from build123d import *

# Parameters (mm, degrees)
SKETCH_1_W                    = 280
SKETCH_1_H                    = 35
EXTRUDE_1_DEPTH               = 26
SKETCH_3_R                    = 9
CUT_EXTRUDE_1_DEPTH           = 36
SKETCH_4_W                    = 25
SKETCH_4_H                    = 26
CUT_EXTRUDE_2_DEPTH           = 1
HOLE_WIZARD_M4_1_D            = 3.3
HOLE_WIZARD_M4_1_DEPTH        = 10.1
HOLE_WIZARD_M4_1_TIP          = 0.991420021
SKETCH_7_W                    = 220
SKETCH_7_H                    = 15
CUT_EXTRUDE_3_DEPTH           = 27
SKETCH_8_W                    = 40
SKETCH_8_H                    = 26
EXTRUDE_2_DEPTH               = 35
SKETCH_15_W                   = 58.430685067
SKETCH_15_H                   = 44.376242578
CUT_EXTRUDE_7_DEPTH           = 3
SKETCH_17_W                   = 40
SKETCH_17_H                   = 26
EXTRUDE_4_DEPTH               = 30
SKETCH_18_W                   = 20
SKETCH_18_H                   = 62
CUT_EXTRUDE_8_DEPTH           = 27
SKETCH_19_W                   = 30
SKETCH_19_H                   = 26
CUT_EXTRUDE_11_DEPTH          = 7
HOLE_WIZARD_M5_1_2_AT_2_COUNT = 2
HOLE_WIZARD_M5_1_2_AT_2_PITCH = 30
CHAMFER_1_SIZE                = 5
CHAMFER_1_SIZE2               = 2.886751346
CHAMFER_2_SIZE                = 5
CHAMFER_2_SIZE2               = 2.886751346
SKETCH_25_R                   = 2.5
CUT_EXTRUDE_12_DEPTH          = 21.0000001
SKETCH_26_R                   = 2.5
CUT_EXTRUDE_13_DEPTH          = 161.0000001
SKETCH_27_R                   = 5
CUT_EXTRUDE_14_DEPTH          = 83
SKETCH_28_R                   = 7
CUT_EXTRUDE_15_DEPTH          = 6
SKETCH_31_W                   = 13
SKETCH_31_H                   = 28
CUT_EXTRUDE_16_DEPTH          = 1
HOLE_WIZARD_M3_1_D            = 2.5
HOLE_WIZARD_M3_1_DEPTH        = 7.5
HOLE_WIZARD_M3_1_TIP          = 0.751075774
SKETCH_34_W                   = 5
SKETCH_34_H                   = 8
CUT_EXTRUDE_17_DEPTH          = 27


with BuildPart() as part:
    # 草图1 → 凸台-拉伸1 (new body)
    with BuildSketch(Plane.XY):
        with Locations((140, 17.5)):
            Rectangle(SKETCH_1_W, SKETCH_1_H)
    extrude(amount=EXTRUDE_1_DEPTH)

    # 草图3 → 切除-拉伸1 (cut, through all)
    with BuildSketch(Plane.XZ):
        with Locations((17, 13)):
            Circle(SKETCH_3_R)
        with Locations((263, 13)):
            Circle(SKETCH_3_R)
    extrude(amount=-CUT_EXTRUDE_1_DEPTH, mode=Mode.SUBTRACT)

    # 草图4 → 切除-拉伸2 (cut)
    with BuildSketch(Plane(origin=(0, 35, 0), x_dir=(1, 0, 0), z_dir=(0, 1, 0))):
        with Locations((140, -13)):
            Rectangle(SKETCH_4_W, SKETCH_4_H)
    extrude(amount=-CUT_EXTRUDE_2_DEPTH, mode=Mode.SUBTRACT)

    # M4 螺纹孔1
    with Locations(Plane(origin=(0, 34, 0), x_dir=(1, 0, 0), z_dir=(0, 1, 0))):
        with Locations((146, -21.5), (134, -21.5), (146, -4.5), (133.546958493, -4.5)):
            Hole(HOLE_WIZARD_M4_1_D / 2, depth=HOLE_WIZARD_M4_1_DEPTH)
            with Locations((0, 0, -(HOLE_WIZARD_M4_1_DEPTH + HOLE_WIZARD_M4_1_TIP / 2))):  # 118° drill point
                Cone(0, HOLE_WIZARD_M4_1_D / 2, HOLE_WIZARD_M4_1_TIP, mode=Mode.SUBTRACT)

    # 草图7 → 切除-拉伸3 (cut, through all)
    with BuildSketch(Plane.XY.offset(26)):
        with Locations((140, 7.5)):
            Rectangle(SKETCH_7_W, SKETCH_7_H)
    extrude(amount=-CUT_EXTRUDE_3_DEPTH, mode=Mode.SUBTRACT)

    # 草图8 → 凸台-拉伸2 (add)
    with BuildSketch(Plane.XZ.offset(-15)):
        with Locations((140, 13)):
            Rectangle(SKETCH_8_W, SKETCH_8_H)
    extrude(amount=EXTRUDE_2_DEPTH)

    # 草图15 → 切除-拉伸7 (cut)
    with BuildSketch(Plane.XZ.offset(20)):
        with Locations((130.784657466, 3.811878711)):
            Rectangle(SKETCH_15_W, SKETCH_15_H)
    extrude(amount=-CUT_EXTRUDE_7_DEPTH, mode=Mode.SUBTRACT)

    # 草图17 → 凸台-拉伸4 (add)
    with BuildSketch(Plane.XZ.offset(17)):
        with Locations((140, 13)):
            Rectangle(SKETCH_17_W, SKETCH_17_H)
    extrude(amount=EXTRUDE_4_DEPTH)

    # 草图18 → 切除-拉伸8 (cut, through all)
    with BuildSketch(Plane(origin=(0, 0, 0), x_dir=(-1, 0, 0), z_dir=(0, 0, -1))):
        with Locations((-140, -16)):
            Rectangle(SKETCH_18_W, SKETCH_18_H)
    extrude(amount=-CUT_EXTRUDE_8_DEPTH, mode=Mode.SUBTRACT)

    # 草图19 → 切除-拉伸11 (cut)
    with BuildSketch(Plane.XZ):
        with Locations((265, 13)):
            Rectangle(SKETCH_19_W, SKETCH_19_H)
        with Locations((15, 13)):
            Rectangle(SKETCH_19_W, SKETCH_19_H)
    extrude(amount=-CUT_EXTRUDE_11_DEPTH, mode=Mode.SUBTRACT)

    # 草图21 → Hole Wizard M5 _1 (revolve, cut)
    with BuildSketch(Plane(origin=(280, 21, 13), x_dir=(0, 0, -1), z_dir=(0, 1, 0))):
        Polygon((0, 0), (0, 13.6618073), (2.1, 12.4), (2.1, 0), align=None)
    hole_wizard_m5_1 = revolve(axis=Axis((286.35, 21, 13), (-1, 0, 0)), mode=Mode.SUBTRACT)

    # 镜向1: Hole Wizard M5 _1 across plane
    add(hole_wizard_m5_1.mirror(Plane.ZY.offset(-140)), mode=Mode.SUBTRACT)

    # 草图24 → Hole Wizard M5 _1 2 (revolve, cut)
    with BuildSketch(Plane(origin=(160, -35, 10), x_dir=(0, 0, -1), z_dir=(0, 1, 0))):
        Polygon((0, 0), (0, 14.052366702), (2.75, 12.4), (2.75, 5.4), (5, 5.4), (5, 0), align=None)
    hole_wizard_m5_1_2 = revolve(axis=Axis((166.35, -35, 10), (-1, 0, 0)), mode=Mode.SUBTRACT)

    # Hole Wizard M5 _1 2 at 2: Hole Wizard M5 _1 2 ×2
    with Locations(*[(0, i * HOLE_WIZARD_M5_1_2_AT_2_PITCH, 0) for i in range(1, HOLE_WIZARD_M5_1_2_AT_2_COUNT)]):
        add(hole_wizard_m5_1_2, mode=Mode.SUBTRACT)

    # 倒角1
    chamfer_1_edges = [part.edges().sort_by_distance(p)[0] for p in [
        (150, -16, 0),
    ]]
    chamfer_1_side = [part.faces().sort_by_distance(p)[0] for p in [
        (150, -15.878511748, 13.091116189),
    ]]
    chamfer(chamfer_1_edges, length=CHAMFER_1_SIZE, length2=CHAMFER_1_SIZE2, reference=chamfer_1_side[0])

    # 倒角2
    chamfer_2_edges = [part.edges().sort_by_distance(p)[0] for p in [
        (130, -16, 0),
    ]]
    chamfer_2_side = [part.faces().sort_by_distance(p)[0] for p in [
        (130, -16, 13),
    ]]
    chamfer(chamfer_2_edges, length=CHAMFER_2_SIZE, length2=CHAMFER_2_SIZE2, reference=chamfer_2_side[0])

    # 镜向2: Hole Wizard M5 _1 2 across plane
    add(hole_wizard_m5_1_2.mirror(Plane.ZY.offset(-140)), mode=Mode.SUBTRACT)

    # 镜向2 copy 1 sketch → 镜向2 copy 1 (revolve, cut)
    with BuildSketch(Plane(origin=(120, -5, 10), x_dir=(0, 0, -1), z_dir=(0, 1, 0))):
        Polygon((0, 0), (0, -14.052366702), (2.75, -12.4), (2.75, -5.4), (5, -5.4), (5, 0), align=None)
    revolve(axis=Axis((113.65, -5, 10), (-1, 0, 0)), mode=Mode.SUBTRACT)

    # 草图25 → 切除-拉伸12 (cut, through all)
    with BuildSketch(Plane.XZ.offset(-15)):
        with Locations((140, 20.49725583)):
            Circle(SKETCH_25_R)
    extrude(amount=-CUT_EXTRUDE_12_DEPTH, mode=Mode.SUBTRACT)

    # 草图26 → 切除-拉伸13 (cut, through all)
    with BuildSketch(Plane.ZY.offset(-120)):
        with Locations((10, -20)):
            Circle(SKETCH_26_R)
    extrude(amount=-CUT_EXTRUDE_13_DEPTH, mode=Mode.SUBTRACT)

    # 草图27 → 切除-拉伸14 (cut, through all)
    with BuildSketch(Plane(origin=(0, 35, 0), x_dir=(1, 0, 0), z_dir=(0, 1, 0))):
        with Locations((196.4, -13)):
            Circle(SKETCH_27_R)
        with Locations((83.6, -13)):
            Circle(SKETCH_27_R)
    extrude(amount=-CUT_EXTRUDE_14_DEPTH, mode=Mode.SUBTRACT)

    # 草图28 → 切除-拉伸15 (cut)
    with BuildSketch(Plane(origin=(0, 35, 0), x_dir=(1, 0, 0), z_dir=(0, 1, 0))):
        with Locations((196.4, -13)):
            Circle(SKETCH_28_R)
        with Locations((83.6, -13)):
            Circle(SKETCH_28_R)
    extrude(amount=-CUT_EXTRUDE_15_DEPTH, mode=Mode.SUBTRACT)

    # 草图31 → 切除-拉伸16 (cut)
    with BuildSketch(Plane.XY.offset(26)):
        with Locations((16.4, 21)):
            Rectangle(SKETCH_31_W, SKETCH_31_H)
    extrude(amount=-CUT_EXTRUDE_16_DEPTH, mode=Mode.SUBTRACT)

    # M3 螺纹孔1
    with Locations(Plane.XY.offset(25)):
        with Locations((17.9, 12), (17.9, 22)):
            Hole(HOLE_WIZARD_M3_1_D / 2, depth=HOLE_WIZARD_M3_1_DEPTH)
            with Locations((0, 0, -(HOLE_WIZARD_M3_1_DEPTH + HOLE_WIZARD_M3_1_TIP / 2))):  # 118° drill point
                Cone(0, HOLE_WIZARD_M3_1_D / 2, HOLE_WIZARD_M3_1_TIP, mode=Mode.SUBTRACT)

    # 草图34 → 切除-拉伸17 (cut, through all)
    with BuildSketch(Plane.XY.offset(26)):
        with Locations((2.5, 31)):
            Rectangle(SKETCH_34_W, SKETCH_34_H)
    extrude(amount=-CUT_EXTRUDE_17_DEPTH, mode=Mode.SUBTRACT)


solid = part.part
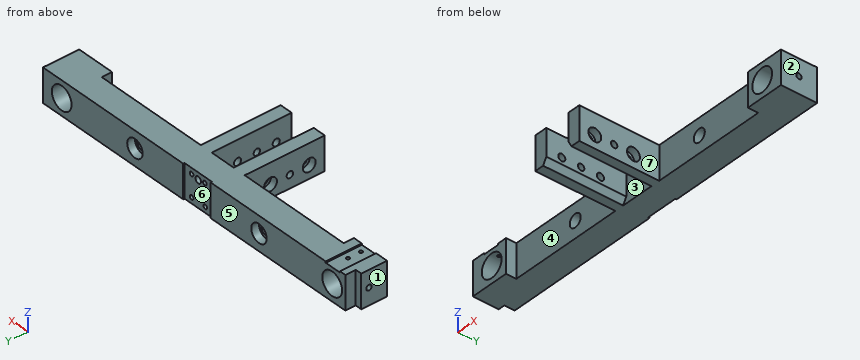
The model under review builds one solid part; all positions refer to its coordinate system, in mm. Face numbers are marked on the shaded views. A direction names the side the tool comes from. Give positions to 0.01 mm unless a question says otherwise; leave off trailing zeros. Loops run counter-clockwise (first coordinate to the right, second up) from the corner with the lowest first, then second, coordinate; pieces in that order, holes last. Notation, with made-up numbers: (5.25, 8.5) -> (10.25, 8.5) arc R15 cw to (10.25, 31.5) -> close; hole circle Ø3 at (14, 15). An arc over 180 degrees is marked (long way). Answer as a JSON object with one key per item and string values. Group by question number.
Q1. Take a section at B-B (x = 140). Write out the cut boundary in (y, z), plus the area to 3 significant figures.
Q2. Take a section at A-A (y = -35). Write out the cut boundary in (x, z), plus the area to 3 significant figures.
Q3. Draft analysis for pull direction X (two halves, no side actions). For the marked faces 1, 2, 3 and 4, state which applies: pulls with the +X half, pulls with the -X half, needs draft (parallel to the pull), parting line crosses it, or undercut.
Q4. Take a section at D-D (x = 196.4). Write out the cut boundary in (y, z), plus the area to 3 significant figures.
Q5. Wall thickness on line 1 along X through (y, z) = (-40, 17.75); line 2 along Z through (x, y) = (84, 20); line 3 along Y through (x, z) = (3.75, 13): over which ranges is each line inside the solid? List them lowest first.
Q6. Tool access review of the marked faces 5, 6 and 7: name each direction out of +Z, -Z, +X, -X, +Y, -Y from which nothing blocks a thin tool from reaching the whole face with its end or side.
Q7. Insertion check: pin 1 (6 mm diameter, centred on x = 139.5, z = 5, fed in from +Y); pin 2 (6 mm diameter, centred on y = -20, z = 4, fed in from +X); pin 3 (3 mm diameter, centred on x = 190.5, z = 16.5, fed in from -Y). Each pin has a flat end and moves straight along its axis. Give the tip position at first contact, or say it passes through.
Q8. Take a section at C-C (y = 4.5). Write out the cut boundary in (x, z), plus the area to 3 significant figures.
Answer below:
{
 "1": {"outline": "(15, 0) -> (34, 0) -> (34, 18) -> (15, 18) -> close; (15, 23) -> (34, 23) -> (34, 26) -> (15, 26) -> close", "area": "399 mm2"},
 "2": {"outline": "(120, 0) -> (127.11, 0) -> (130, 5) -> (130, 7.25) -> (125.4, 7.25) -> (125.4, 5) -> (120, 5) -> close; (120, 15) -> (125.4, 15) -> (125.4, 12.75) -> (130, 12.75) -> (130, 26) -> (120, 26) -> close; (150, 5) -> (152.89, 0) -> (160, 0) -> (160, 5) -> (154.6, 5) -> (154.6, 7.25) -> (150, 7.25) -> close; (150, 12.75) -> (154.6, 12.75) -> (154.6, 15) -> (160, 15) -> (160, 26) -> (150, 26) -> close", "area": "347 mm2"},
 "3": {"face 1": "pulls with the -X half", "face 2": "pulls with the +X half", "face 3": "undercut", "face 4": "undercut"},
 "4": {"outline": "(15, 0) -> (35, 0) -> (35, 6) -> (29, 6) -> (29, 8) -> (15, 8) -> close; (15, 18) -> (29, 18) -> (29, 20) -> (35, 20) -> (35, 26) -> (15, 26) -> close", "area": "296 mm2"},
 "5": {"line 1": "x = 120 to 130, 150 to 160", "line 2": "z = 0 to 8.02, 17.98 to 26", "line 3": "y = 7 to 18.9, 23.1 to 27"},
 "6": {"face 5": "+Z, -Z, +X, -X, +Y", "face 6": "+Z, -Z, +Y", "face 7": "+Z, -Z, -Y"},
 "7": {"pin 1": "stops at y = 34", "pin 2": "stops at x = 160", "pin 3": "stops at y = 15"},
 "8": {"outline": "(120, 0) -> (127.11, 0) -> (130, 5) -> (130, 26) -> (120, 26) -> close; (150, 5) -> (152.89, 0) -> (160, 0) -> (160, 26) -> (150, 26) -> close", "area": "506 mm2"}
}
